The listing builds one solid part. Answer for the finished solid, in the listing's coordinates (mm). Coordinates: 2 decimals unless noted, no trailing zeros. Loops run counter-clockwise (first coordinate to the right, second up) from the corner with the lowest first, then second, coordinate; pieces in that order, holes last. Notation, with made-up numbers: M -23,37.25 L 0,37.25 A20 cw 0,42.25 Z; hole C 22.25,34.25 d6. An arc over 180 degrees is marked long. Answer in a Markdown table with one row per item. Add a question column.
from build123d import *

# Parameters (mm, degrees)
F0_W     = 300
F0_H     = 200
F0_R     = 15
F1_DEPTH = 100
F2_R     = 25
F3_R     = 25


with BuildPart() as f1:
    # F0 (on Top) → F1 (new body)
    with BuildSketch(Plane.XY):
        with Locations((7.243371, 7.086681)):
            Rectangle(F0_W, F0_H)
        with Locations((115.392633, 0)):
            Circle(F0_R, mode=Mode.SUBTRACT)
    extrude(amount=F1_DEPTH)

    # F2
    f2_edges = [f1.edges().sort_by_distance(p)[0] for p in [
        (157.243371, 107.086681, 50),
    ]]
    fillet(f2_edges, radius=F2_R)

    # F3
    f3_edges = [f1.edges().sort_by_distance(p)[0] for p in [
        (-142.756629, 107.086681, 50),
        (-142.756629, -92.913319, 50),
        (157.243371, -92.913319, 50),
    ]]
    fillet(f3_edges, radius=F3_R)


solid = f1.part
(1) A cutting plane is placed at B-B (z = 70.5). Give the vertices of the cut face in (x, y), plus the area to 3 significant figures.
(2) The mould has two halves that part along X. Classify faces 1 (the face through (5, -92.913, 49)), 2 (the face through (157.243, 6, 49)), 3 (the face through (100.407, 0.66, 49.3)): released by +X, released by -X, zero draft, split by the parting line, or undercut.
(3) A cutting plane is placed at A-A (y = 0). Give the vertices of the cut face in (x, z), plus the area to 3 significant figures.
(4) Straight lines are drawn through the part: line 1 (Y direction, x = 119.5, z = 10); line 2 (X direction, y = 8, z = 46.5); line 3 (X direction, y = 99, z = 14). For each, find the intervals that lie inside material, in ascending order.
(5) This flat-tipped pin is pushed along its axis until it touches: pin 1 (4 mm diameter, centred on x = -26, y = 27.5, fed in from -Z). Where does it stop, or does it pass through?
Solved:
| question | item | result |
|---|---|---|
| 1 | outline | M -142.76,-67.91 A25 ccw -117.76,-92.91 L 132.24,-92.91 A25 ccw 157.24,-67.91 L 157.24,82.09 A25 ccw 132.24,107.09 L -117.76,107.09 A25 ccw -142.76,82.09 Z; hole C 115.39,0 d30 |
| 1 | area | 58,800 mm² |
| 2 | face 1 | zero draft |
| 2 | face 2 | released by +X |
| 2 | face 3 | undercut |
| 3 | outline | M -142.76,0 L 100.39,0 L 100.39,100 L -142.76,100 Z; M 130.39,0 L 157.24,0 L 157.24,100 L 130.39,100 Z |
| 3 | area | 27,000 mm² |
| 4 | line 1 | y = -92.91 to -14.43, 14.43 to 107.09 |
| 4 | line 2 | x = -142.76 to 102.7, 128.08 to 157.24 |
| 4 | line 3 | x = -136.17 to 150.65 |
| 5 | pin 1 | stops at z = 0 |
